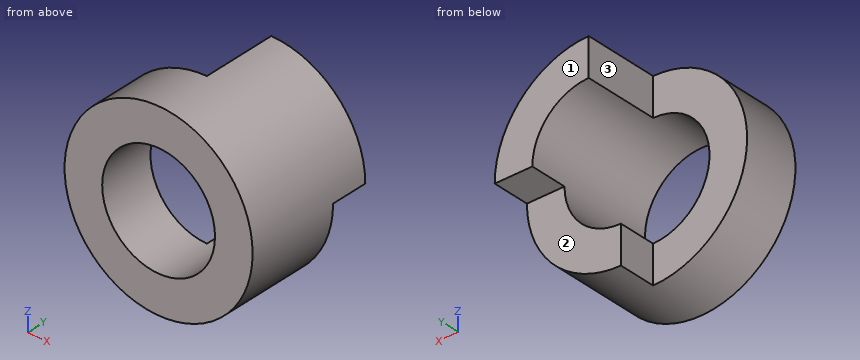
```python
from build123d import *

# Parameters (mm, degrees)
SKETCH1_R           = 5
SKETCH1_R_2         = 3
BOSS_EXTRUDE1_DEPTH = 7
SKETCH3_W           = 6.288888245
SKETCH3_H           = 10.422150442
CUT_EXTRUDE1_DEPTH  = 4
SKETCH4_W           = 5
SKETCH4_H           = 5
CUT_EXTRUDE2_DEPTH  = 2


with BuildPart() as part:
    # Sketch1 → Boss-Extrude1 (new body)
    with BuildSketch(Plane(origin=(0, 0, 0), x_dir=(1, 0, 0), z_dir=(0, 1, 0))):
        Circle(SKETCH1_R)
        Circle(SKETCH1_R_2, mode=Mode.SUBTRACT)
    extrude(amount=BOSS_EXTRUDE1_DEPTH)

    # Sketch3 → Cut-Extrude1 (cut)
    with BuildSketch(Plane(origin=(0, 7, 0), x_dir=(1, 0, 0), z_dir=(0, 1, 0))):
        with Locations((-3.144444123, -0.211075221)):
            Rectangle(SKETCH3_W, SKETCH3_H)
    extrude(amount=-CUT_EXTRUDE1_DEPTH, mode=Mode.SUBTRACT)

    # Sketch4 → Cut-Extrude2 (cut)
    with BuildSketch(Plane(origin=(0, 7, 0), x_dir=(1, 0, 0), z_dir=(0, 1, 0))):
        with Locations((2.5, 2.5)):
            Rectangle(SKETCH4_W, SKETCH4_H)
    extrude(amount=-CUT_EXTRUDE2_DEPTH, mode=Mode.SUBTRACT)


solid = part.part
```
Geometry check sheet. Reference: the model listing, model coordinates, mm. Face numbers are marked on the shaded views. A direction names the side the tool comes from. Give positions to 0.01 mm unless a question says otherwise; leave off trailing zeros. Write each loop counter-clockwise with the first axis right and the second up, starting at its lowest first coordinate (ties: lowest second). Pieces come first, ordered by that corner, then holes. Notation, with made-up numbers: (40.5, 44.25) -> (68.5, 44.25) arc R28 ccw to (68.5, 75.25) -> close; hole circle Ø4 at (-6, 86). An arc over 180 degrees is marked (long way). Use one line per item in the form item = value.
Item 1: Sectioned sample at D-D on x = 3.75. Enter the section's corners in (y, z), plus the area to 3 significant figures.
Results list:
outline = (0, -3.31) -> (5, -3.31) -> (5, 0) -> (7, 0) -> (7, 3.31) -> (0, 3.31) -> close
area = 39.7 mm2
Item 2: Depth check by flat-ended pin: pin 1 Ø5 at (x, z) = (-1, 0) entering from +Y; pin 2 Ø4 at (x, z) = (2.5, -3.5) entering from +Y; pin 3 Ø1.6 at (y, z) = (6, 4) entering from -X. Enter the tip coordinate at first touch or a pass-through.
Results list:
pin_1 = 3
pin_2 = 5
pin_3 = 0
Item 3: Access from +Z, -Z, +X, -X, +Y, -Y to the whole of each face (thin tool, end or side, straight path). Record for the marked faces 1, 2 and 3.
Results list:
face_1 = +Z, -Z, +X, -X, +Y
face_2 = -Z, +X, -X, +Y
face_3 = +Z, -Z, -X, +Y
Item 4: Sectioned sample at A-A on x = -2.25. Enter the section's corners in (y, z), plus the area to 3 significant figures.
Results list:
outline = (0, -4.47) -> (3, -4.47) -> (3, -1.98) -> (0, -1.98) -> close; (0, 1.98) -> (3, 1.98) -> (3, 4.47) -> (0, 4.47) -> close
area = 14.9 mm2
Item 5: Sectioned sample at C-C on y = 1.25. Enter the section's corners in (x, z).
Results list:
outline = circle Ø10 at (0, 0); hole circle Ø6 at (0, 0)
Item 6: Scan lines: line 1 (Z direction, x = 0, y = 1.75); line 2 (X direction, y = 3.25, z = 0). Record each from-to range of solid material in increasing order.
Results list:
line_1 = -5 to -3, 3 to 5
line_2 = 3 to 5
Item 7: Sectioned sample at B-B on z = 0.75. Enter the section's corners in (x, y), plus the area to 3 significant figures.
Results list:
outline = (-4.94, 0) -> (-2.9, 0) -> (-2.9, 3) -> (-4.94, 3) -> close; (2.9, 0) -> (4.94, 0) -> (4.94, 7) -> (2.9, 7) -> close
area = 20.4 mm2
